Geometry: final body of the model. Coordinates: model frame, mm. Face numbers are marked on the shaded views. A direction names the side the tool comes from. Give positions to 0.01 mm unless a question says otherwise; leave off trailing zeros. Order: outer loops, then holes, each group sorted by start corner. A loop starts at its lowest first (then second) coordinate and runs counter-clockwise, first axis right, second up. Notation, with made-up numbers: (30.5, 26) -> (81.5, 26) arc R15 ccw to (81.5, 47) -> close; hole circle Ø6 at (78, -10.75). An arc over 180 degrees is marked (long way). Write item = value, one per line.
```python
from build123d import *

# Parameters (mm, degrees)
SKETCH1_R           = 4.15
BOSS_EXTRUDE1_DEPTH = 50
CUT_EXTRUDE1_DEPTH  = 16
CHAMFER1_SIZE       = 0.5


with BuildPart() as part:
    # Sketch1 → Boss-Extrude1 (new body)
    with BuildSketch(Plane(origin=(0, 0, 0), x_dir=(1, 0, 0), z_dir=(0, 1, 0))):
        Circle(SKETCH1_R)
    extrude(amount=BOSS_EXTRUDE1_DEPTH)

    # Sketch2 → Cut-Extrude1 (cut)
    with BuildSketch(Plane(origin=(0, 50, 0), x_dir=(1, 0, 0), z_dir=(0, 1, 0))):
        with BuildLine():
            Line((-2.701851217, 3.15), (2.701851217, 3.15))
            ThreePointArc((2.701851217, 3.15), (0, 4.15), (-2.701851217, 3.15))
        make_face()
    cut_extrude1 = extrude(amount=-CUT_EXTRUDE1_DEPTH, mode=Mode.SUBTRACT)

    # Mirror1: Cut-Extrude1 across plane
    add(cut_extrude1.mirror(Plane.ZX.offset(25)), mode=Mode.SUBTRACT)

    # Chamfer1
    chamfer1_edges = [part.edges().sort_by_distance(p)[0] for p in [
        (-1.733467255, 0, 3.770622134),
        (-1.733467255, 50, 3.770622134),
    ]]
    chamfer(chamfer1_edges, length=CHAMFER1_SIZE)


solid = part.part
```
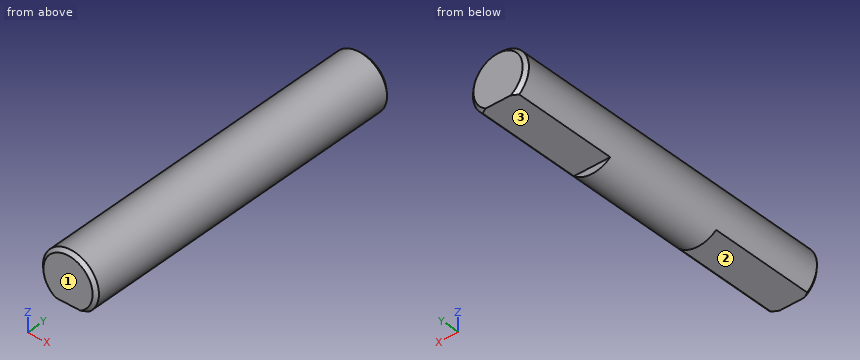
1) Section query A-A (x = 0). Output: boundary loops of the cut face in (y, z), plus the area to 3 significant figures.
Check sheet entries:
outline = (0, -3.15) -> (16, -3.15) -> (16, -4.15) -> (34, -4.15) -> (34, -3.15) -> (50, -3.15) -> (50, 3.65) -> (49.5, 4.15) -> (0.5, 4.15) -> (0, 3.65) -> close
area = 383 mm²
2) First-contact query: P1, Ø1, axis at x = 2.5, y = 17, coming from the -Z side; P2, Ø0.5, axis at x = -1, z = -3.5, coming from the -Y side. Flat tips, straight axial feed; report the tip coordinate or a pass-through.
Check sheet entries:
P1 = -3.64
P2 = 16
3) Section query C-C (y = 46). Output: boundary loops of the cut face in (x, z), plus the area to 3 significant figures.
Check sheet entries:
outline = (-2.7, -3.15) -> (2.7, -3.15) arc R4.15 ccw (long way) to start
area = 50.4 mm²
4) Reachability of the marked faces 1, 2 and 3 from +Z, -Z, +X, -X, +Y, -Y: full face, straight path, thin tool, end or side. Return the list, or none.
Check sheet entries:
face_1 = +Z, -Z, +X, -X, -Y
face_2 = -Z, +X, -X, -Y
face_3 = -Z, +X, -X, +Y
5) Line query: line 1 (X direction, y = 39, z = -0.25); line 2 (Y direction, x = -2.25, z = -3.25); line 3 (X direction, y = 26, z = 3.75). Output: solid intervals per line, ascending. Write a range as from..to.
Check sheet entries:
line_1 = -4.14..4.14
line_2 = 16..34
line_3 = -1.78..1.78
6) Section query B-B (y = 31). Output: boundary loops of the cut face in (x, z).
Check sheet entries:
outline = circle Ø8.3 at (0, 0)
